Verification items for the finished model (mm, model axes). Face numbers are marked on the shaded views. A direction names the side the tool comes from. Give positions to 0.01 mm unless a question says otherwise; leave off trailing zeros. Order: outer loops, then holes, each group sorted by start corner. A loop starts at its lowest first (then second) coordinate and runs counter-clockwise, first axis right, second up. Notation, with made-up numbers: (25, -37.75) -> (84, -37.75) arc R23 cw to (84, -6.75) -> close; hole circle Ø4 at (82.5, 55). An arc over 180 degrees is marked (long way). Write each question's results on one line, items separated by ' | '. Start each with the question number.
1. Set-up check for the marked faces 5 and 6: record each of +Z, -Z, +X, -X, +Y, -Y from which the full face is reachable in a straight line by a thin tool's end or side.
2. Depth check by flat-ended pin: pin 1 Ø0.8 at (x, z) = (59.5, -33.5) entering from +Y; pin 2 Ø3.5 at (y, z) = (41.275, -16.637) entering from +X; pin 3 Ø4 at (x, z) = (-27.5, -33.5) entering from +Y. Enter the tip coordinate at first touch or a pass-through.
3. Material ranges on L1, parallel to X at y = 83.5, z = 34.5; L2, parallel to X at y = 91, z = 34; L3, parallel to Z at x = 71.5, y = 69.5, recorded low to high. Write a range as from..to.
4. Cross-section at B-B, the plane x = 1. Enter the section's corners in (y, z).
5. Cross-section at A-A, the plane z = 0. Enter the section's corners in (x, y).
6. Mould release check, pull along Z, two halves, no side actions. Record for the marked faces 1, 2, 3 and 4: +Z half, -Z half, draft (parallel to the pull), parting line (faces both ways), or undercut.
7. Cross-section at D-D, the plane y = 100.5. Enter the section's corners in (x, z).
8. Cross-section at C-C, the plane y = 68.58. Enter the section's corners in (x, z).
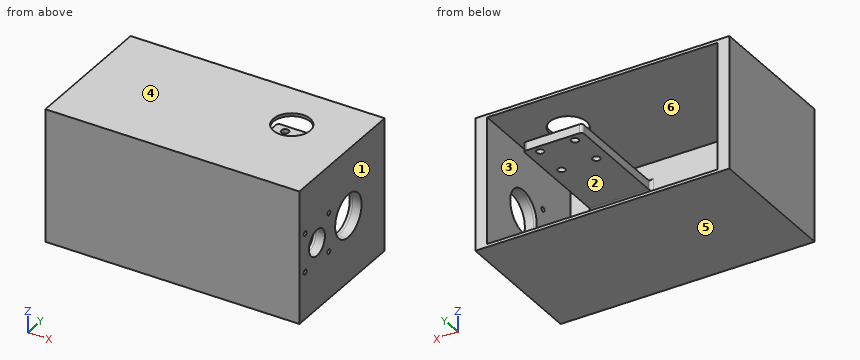
from build123d import *

# Parameters (mm, degrees)
SKETCH1_W           = 203.2
SKETCH1_H           = 114.3
BOSS_EXTRUDE1_DEPTH = 119.38
SHELL1_T            = -2.54
SKETCH2_R           = 18.5
SKETCH2_R_2         = 2.032
SKETCH2_R_3         = 11.176
CUT_EXTRUDE1_DEPTH  = 2.54
SKETCH3_W           = 114.3
SKETCH3_H           = 119.38
SKETCH3_R           = 18.5
SKETCH3_R_2         = 2.032
SKETCH3_R_3         = 11.176
BOSS_EXTRUDE3_DEPTH = 7.62
SKETCH4_R           = 15.875
CUT_EXTRUDE2_DEPTH  = 2.54
SKETCH5_W           = 50.7
SKETCH5_H           = 7.62
BOSS_EXTRUDE4_DEPTH = 95.25
CUT_EXTRUDE3_REACH  = 189.987
SKETCH6_R           = 3.175
FILLET1_R           = 2.54
FILLET2_R           = 2.54
SKETCH7_W           = 114.3
SKETCH7_H           = 119.38
BOSS_EXTRUDE5_DEPTH = 7.62
SKETCH8_R           = 2.54
SKETCH8_R_2         = 1.27
BOSS_EXTRUDE6_DEPTH = 5.08


with BuildPart() as part:
    # Sketch1 → Boss-Extrude1 (new body)
    with BuildSketch(Plane(origin=(0, 0, 0), x_dir=(1, 0, 0), z_dir=(0, 1, 0))):
        Rectangle(SKETCH1_W, SKETCH1_H)
    extrude(amount=BOSS_EXTRUDE1_DEPTH)

    # Shell1
    shell1_openings = [part.faces().sort_by_distance(p)[0] for p in [
        (0, 119.38, 0),
    ]]
    offset(amount=SHELL1_T, openings=shell1_openings, kind=Kind.INTERSECTION)

    # Sketch2 → Cut-Extrude1 (cut)
    with BuildSketch(Plane.ZY.offset(-99.06)):
        with Locations((0, 68.58)):
            Circle(SKETCH2_R)
        with Locations((16.637, 41.275)):
            Circle(SKETCH2_R_2)
        with Locations(Location((16.637, 8.001, 0), (0, 0, 180))):
            Circle(SKETCH2_R_2)
        with Locations((-16.637, 8.001)):
            Circle(SKETCH2_R_2)
        with Locations(Location((-16.637, 41.275, 0), (0, 0, 180))):
            Circle(SKETCH2_R_2)
        with Locations((0, 24.638)):
            Circle(SKETCH2_R_3)
    extrude(amount=-CUT_EXTRUDE1_DEPTH, mode=Mode.SUBTRACT)

    # Sketch3 → Boss-Extrude3 (add)
    with BuildSketch(Plane(origin=(101.6, 0, 0), x_dir=(0, 0, -1), z_dir=(1, 0, 0))):
        with Locations((0, 59.69)):
            Rectangle(SKETCH3_W, SKETCH3_H)
        with Locations(Location((0, 68.58, 0), (0, 0, 180))):
            Circle(SKETCH3_R, mode=Mode.SUBTRACT)
        with Locations((-16.637, 8.001)):
            Circle(SKETCH3_R_2, mode=Mode.SUBTRACT)
        with Locations(Location((16.637, 8.001, 0), (0, 0, 180))):
            Circle(SKETCH3_R_2, mode=Mode.SUBTRACT)
        with Locations((16.637, 41.275)):
            Circle(SKETCH3_R_2, mode=Mode.SUBTRACT)
        with Locations(Location((-16.637, 41.275, 0), (0, 0, 180))):
            Circle(SKETCH3_R_2, mode=Mode.SUBTRACT)
        with Locations(Location((0, 24.638, 0), (0, 0, 180))):
            Circle(SKETCH3_R_3, mode=Mode.SUBTRACT)
    extrude(amount=BOSS_EXTRUDE3_DEPTH)

    # Sketch4 → Cut-Extrude2 (cut)
    with BuildSketch(Plane.XY.offset(57.15)):
        with Locations((55.88, 76.2)):
            Circle(SKETCH4_R)
    extrude(amount=-CUT_EXTRUDE2_DEPTH, mode=Mode.SUBTRACT)

    # Sketch5 → Boss-Extrude4 (add)
    with BuildSketch(Plane(origin=(0, 2.54, 0), x_dir=(1, 0, 0), z_dir=(0, 1, 0))):
        with Locations((55.88, -34.74)):
            Rectangle(SKETCH5_W, SKETCH5_H)
    extrude(amount=BOSS_EXTRUDE4_DEPTH)

    # Sketch6 → Cut-Extrude3 (cut, up to next)
    with BuildSketch(Plane.XY.offset(38.55), mode=Mode.PRIVATE) as cut_extrude3_sk1:
        with Locations((40.88, 91.2)):
            Circle(SKETCH6_R)
    cut_extrude3_tool1 = extrude(cut_extrude3_sk1.sketch, amount=-CUT_EXTRUDE3_REACH, mode=Mode.PRIVATE) & part.part
    # Sketch6 → Cut-Extrude3 (cut, up to next)
    with BuildSketch(Plane.XY.offset(38.55), mode=Mode.PRIVATE) as cut_extrude3_sk2:
        with Locations((70.88, 61.2)):
            Circle(SKETCH6_R)
    cut_extrude3_tool2 = extrude(cut_extrude3_sk2.sketch, amount=-CUT_EXTRUDE3_REACH, mode=Mode.PRIVATE) & part.part
    # Sketch6 → Cut-Extrude3 (cut, up to next)
    with BuildSketch(Plane.XY.offset(38.55), mode=Mode.PRIVATE) as cut_extrude3_sk3:
        with Locations((40.88, 61.2)):
            Circle(SKETCH6_R)
    cut_extrude3_tool3 = extrude(cut_extrude3_sk3.sketch, amount=-CUT_EXTRUDE3_REACH, mode=Mode.PRIVATE) & part.part
    # Sketch6 → Cut-Extrude3 (cut, up to next)
    with BuildSketch(Plane.XY.offset(38.55), mode=Mode.PRIVATE) as cut_extrude3_sk4:
        with Locations((70.88, 91.2)):
            Circle(SKETCH6_R)
    cut_extrude3_tool4 = extrude(cut_extrude3_sk4.sketch, amount=-CUT_EXTRUDE3_REACH, mode=Mode.PRIVATE) & part.part
    add(cut_extrude3_tool1.solids().sort_by_distance((40.88, 91.2, 38.55))[0], mode=Mode.SUBTRACT)
    add(cut_extrude3_tool2.solids().sort_by_distance((70.88, 61.2, 38.55))[0], mode=Mode.SUBTRACT)
    add(cut_extrude3_tool3.solids().sort_by_distance((40.88, 61.2, 38.55))[0], mode=Mode.SUBTRACT)
    add(cut_extrude3_tool4.solids().sort_by_distance((70.88, 91.2, 38.55))[0], mode=Mode.SUBTRACT)

    # Fillet1
    fillet1_edges = [part.edges().sort_by_distance(p)[0] for p in [
        (30.53, 97.79, 34.74),
        (81.23, 97.79, 34.74),
    ]]
    fillet(fillet1_edges, radius=FILLET1_R)

    # Fillet2
    fillet2_edges = [part.edges().sort_by_distance(p)[0] for p in [
        (30.53, 2.54, 34.74),
        (55.88, 2.54, 38.55),
        (81.23, 2.54, 34.74),
        (55.88, 2.54, 30.93),
    ]]
    fillet(fillet2_edges, radius=FILLET2_R)

    # Sketch7 → Boss-Extrude5 (add)
    with BuildSketch(Plane.ZY.offset(101.6)):
        with Locations((0, 59.69)):
            Rectangle(SKETCH7_W, SKETCH7_H)
    extrude(amount=BOSS_EXTRUDE5_DEPTH)

    # Sketch8 → Boss-Extrude6 (add)
    # profile 1 of 4: a face of its own
    with BuildSketch(Plane(origin=(0, 2.54, 0), x_dir=(1, 0, 0), z_dir=(0, 1, 0))):
        with Locations(Location((57.72714395, -23.731482064, 0), (0, 0, 90))):
            Circle(SKETCH8_R)
        with Locations(Location((57.72714395, -23.731482064, 0), (0, 0, 270))):
            Circle(SKETCH8_R_2, mode=Mode.SUBTRACT)
    # profile 2 of 4: a face of its own
    with BuildSketch(Plane(origin=(0, 2.54, 0), x_dir=(1, 0, 0), z_dir=(0, 1, 0))):
        with Locations(Location((59.40714395, 34.233185903, 0), (0, 0, 90))):
            Circle(SKETCH8_R)
        with Locations(Location((59.40714395, 34.233185903, 0), (0, 0, 270))):
            Circle(SKETCH8_R_2, mode=Mode.SUBTRACT)
    # profile 3 of 4: a face of its own
    with BuildSketch(Plane(origin=(0, 2.54, 0), x_dir=(1, 0, 0), z_dir=(0, 1, 0))):
        with Locations(Location((-26.48785605, 34.233185903, 0), (0, 0, 90))):
            Circle(SKETCH8_R)
        with Locations(Location((-26.48785605, 34.233185903, 0), (0, 0, 270))):
            Circle(SKETCH8_R_2, mode=Mode.SUBTRACT)
    # profile 4 of 4: a face of its own
    with BuildSketch(Plane(origin=(0, 2.54, 0), x_dir=(1, 0, 0), z_dir=(0, 1, 0))):
        with Locations(Location((-28.27285605, -23.731482064, 0), (0, 0, 90))):
            Circle(SKETCH8_R)
        with Locations(Location((-28.27285605, -23.731482064, 0), (0, 0, 270))):
            Circle(SKETCH8_R_2, mode=Mode.SUBTRACT)
    extrude(amount=BOSS_EXTRUDE6_DEPTH)


solid = part.part
Results below:
1) face 5: -Z, +X, -X, +Y, -Y | face 6: +Y
2) pin 1: stops at y = 2.54 | pin 2: stops at x = -99.06 | pin 3: stops at y = 7.62
3) L1: x = -109.22..-99.06, 30.53..81.23, 99.06..109.22 | L2: x = -109.22..-99.06, 30.53..37.71, 44.05..67.71, 74.05..81.23, 99.06..109.22 | L3: z = -57.15..-54.61, 30.93..38.55, 54.61..57.15
4) outline: (0, -57.15) -> (119.38, -57.15) -> (119.38, -54.61) -> (2.54, -54.61) -> (2.54, 54.61) -> (119.38, 54.61) -> (119.38, 57.15) -> (0, 57.15) -> close
5) outline: (-109.22, 0) -> (109.22, 0) -> (109.22, 13.46) -> (99.06, 13.46) -> (99.06, 2.54) -> (-99.06, 2.54) -> (-99.06, 119.38) -> (-109.22, 119.38) -> close; (99.06, 35.81) -> (109.22, 35.81) -> (109.22, 50.08) -> (99.06, 50.08) -> close; (99.06, 87.08) -> (109.22, 87.08) -> (109.22, 119.38) -> (99.06, 119.38) -> close
6) face 1: draft | face 2: undercut | face 3: undercut | face 4: +Z half
7) outline: (-109.22, -57.15) -> (109.22, -57.15) -> (109.22, 57.15) -> (-109.22, 57.15) -> close; hole (-99.06, -54.61) -> (99.06, -54.61) -> (99.06, 54.61) -> (-99.06, 54.61) -> close
8) outline: (-109.22, -57.15) -> (109.22, -57.15) -> (109.22, -18.5) -> (99.06, -18.5) -> (99.06, -54.61) -> (-99.06, -54.61) -> (-99.06, 54.61) -> (41.95, 54.61) -> (41.95, 57.15) -> (-109.22, 57.15) -> close; (30.53, 30.93) -> (81.23, 30.93) -> (81.23, 38.55) -> (30.53, 38.55) -> close; (69.81, 54.61) -> (99.06, 54.61) -> (99.06, 18.5) -> (109.22, 18.5) -> (109.22, 57.15) -> (69.81, 57.15) -> close
